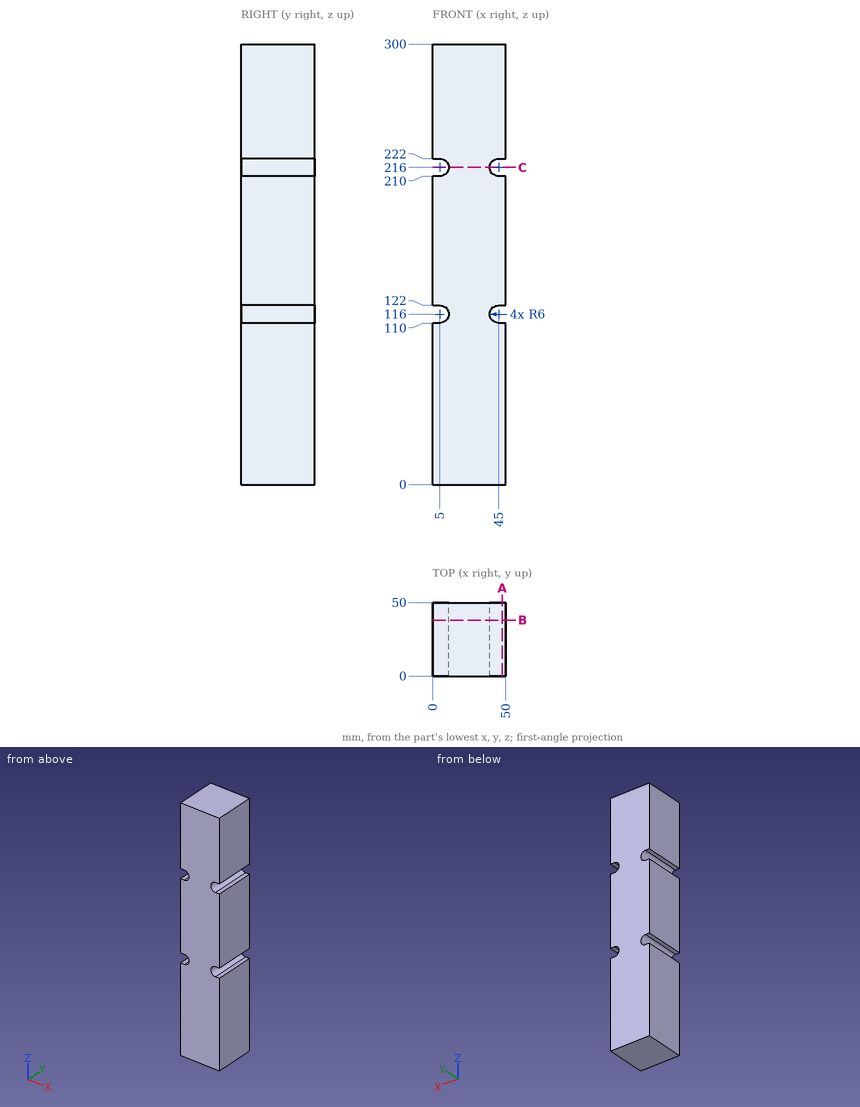
Geometry check sheet. Reference: drawing and pictorial views, mm from the part's lowest x, y, z. Round coordinates to 2 decimals unless told otherwise and drop trailing zeros. Loops run counter-clockwise (first coordinate to the right, second up) from the corner with the lowest first, then second, coordinate; pieces in that order, holes last.
1. Gauge pin test, flat end, axial feed: pin 1 Ø4 at (x, y) = (2.5, 15) entering from -Z. Record the tip position at first contact, or that the pin passes through.
2. Sectioned sample at C-C on z = 216. Record the boundary of the cut face in (x, y).
3. Scan lines: probe 1 along Z at (x, y) = (3, 48.5); probe 2 along Z at (x, y) = (42.5, 44.5); probe 3 along X at (y, z) = (48, 214). Record each from-to range of solid material in increasing order.
4. Sectioned sample at B-B on y = 38. Record the boundary of the cut face in (x, z), and give its area (3 significant figures).
5. Sectioned sample at A-A on x = 47.5. Record the boundary of the cut face in (y, z), and give its area (3 significant figures).
Recorded:
1. pin 1: stops at z = 0
2. outline: (11, 0) - (39, 0) - (39, 50) - (11, 50) - close
3. probe 1: z = 0 to 110, 122 to 210, 222 to 300
3. probe 2: z = 0 to 110.55, 121.45 to 210.55, 221.45 to 300
3. probe 3: x = 10.66 to 39.34
4. outline: (0, 0) - (50, 0) - (50, 110) - (45, 110) arc R6 cw to (45, 122) - (50, 122) - (50, 210) - (45, 210) arc R6 cw to (45, 222) - (50, 222) - (50, 300) - (0, 300) - (0, 222) - (5, 222) arc R6 cw to (5, 210) - (0, 210) - (0, 122) - (5, 122) arc R6 cw to (5, 110) - (0, 110) - close
4. area: 14,500 mm2
5. outline: (0, 0) - (50, 0) - (50, 110) - (0, 110) - close; (0, 122) - (50, 122) - (50, 210) - (0, 210) - close; (0, 222) - (50, 222) - (50, 300) - (0, 300) - close
5. area: 13,800 mm2
